Build history of the part. All positions in model axes, mm. Face numbers are marked on the shaded views. A direction names the side the tool comes from. Coordinates: 2 decimals unless noted, no trailing zeros. Order: outer loops, then holes, each group sorted by start corner. A loop starts at its lowest first (then second) coordinate and runs counter-clockwise, first axis right, second up. Notation, with made-up numbers: M 31,21.5 L 80,21.5 A12 cw 80,26.5 Z; hole C 27,87 d9. An arc over 180 degrees is marked long. Write item = value, one per line. Start each with the question number.
Q1. Band-saw the part on D-D on z = -35. Write the cut outline in (x, y), plus the area to 3 significant figures.
Q2. Band-saw the part on A-A on z = 0. Write the cut outline in (x, y), plus the area to 3 significant figures.
Q3. Pin check, flat tips, straight feed: P1, Ø5, axis at x = -102.5, z = 0, coming from the +Y side; P2, Ø1, axis at x = -105, y = -36, coming from the -Z side; P3, Ø6, axis at x = -121.5, y = -16.5, coming from the +Z side. Stop position of each tip, or through.
Q4. Drill centre lines: probe 1 along Y at (x, z) = (-73.5, 0); probe 2 along Y at (x, z) = (-113, 0); probe 3 along X at (y, z) = (-11, -49.5). Where is each one in solid material? Low to high.
Q5. Band-saw the part on B-B on y = 0. Write the cut outline in (x, z).
Q6. Pull direction Y, two halves, no side cores. Call the marked faces 1, 2 and 3: released by +Y, released by -Y, zero draft, split by the parting line, or undercut.
Q7. 3-axis set-ups, long thin cutter, end or side, ignore diameter. For the marked faces 4 and 5: which of +Z, -Z, +X, -X, +Y, -Y reach the whole face in a straight line?
Q8. Band-saw the part on C-C on x = -163. Write the cut outline in (y, z).
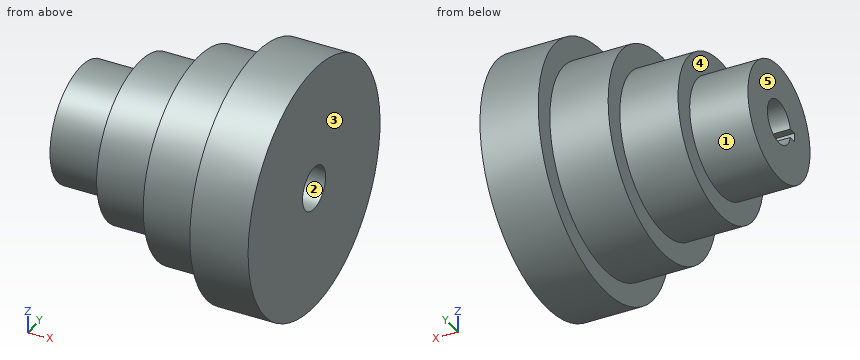
```python
from build123d import *

# Parameters (mm, degrees)
SKETCH2_W          = 6
SKETCH2_H          = 10
CUT_EXTRUDE3_DEPTH = 100


with BuildPart() as part:
    # Sketch1 → Revolve2 (revolve)
    with BuildSketch(Plane.XY, mode=Mode.PRIVATE) as revolve2_sk:
        Polygon((-45.142857143, 22.857142857), (-176, 22.857142857), (-176, 14.867713129), (-16, 14.867713129), (-16, 22.857142857), align=None)
        Polygon((-136, 40), (-176, 40), (-176, 22.857142857), (-45.142857143, 22.857142857), (-45.142857143, 37.142857143), (-128, 37.142857143), (-128, 47), (-88, 47), (-88, 62), (-48, 62), (-48, 77), (-16, 77), (-16, 85), (-56, 85), (-56, 70), (-96, 70), (-96, 55), (-136, 55), align=None)
        Polygon((-45.142857143, 37.142857143), (-45.142857143, 22.857142857), (-16, 22.857142857), (-16, 77), (-48, 77), (-48, 62), (-88, 62), (-88, 47), (-128, 47), (-128, 37.142857143), align=None)
    revolve(revolve2_sk.sketch.rotate(Axis((-176, 0, 0), (1, 0, 0)), 90), axis=Axis((-176, 0, 0), (1, 0, 0)))

    # Sketch2 → Cut-Extrude3 (cut)
    with BuildSketch(Plane.ZY.offset(176)):
        with Locations((0, -14.867713129)):
            Rectangle(SKETCH2_W, SKETCH2_H)
    extrude(amount=-CUT_EXTRUDE3_DEPTH, mode=Mode.SUBTRACT)


solid = part.part
```
Recorded:
q1.outline = M -176,-19.36 L -136,-19.36 L -136,-42.43 L -96,-42.43 L -96,-60.62 L -56,-60.62 L -56,-77.46 L -16,-77.46 L -16,77.46 L -56,77.46 L -56,60.62 L -96,60.62 L -96,42.43 L -136,42.43 L -136,19.36 L -176,19.36 Z
q1.area = 16,000 mm2
q2.outline = M -176,-40 L -136,-40 L -136,-55 L -96,-55 L -96,-70 L -56,-70 L -56,-85 L -16,-85 L -16,-14.87 L -76,-14.87 L -76,-19.87 L -176,-19.87 Z; M -176,14.87 L -16,14.87 L -16,85 L -56,85 L -56,70 L -96,70 L -96,55 L -136,55 L -136,40 L -176,40 Z
q2.area = 14,700 mm2
q3.P1 = 55
q3.P2 = -42.01
q3.P3 = 53.32
q4.probe_1 = -70 to -14.87, 14.87 to 70
q4.probe_2 = -55 to -19.87, 14.87 to 55
q4.probe_3 = -136 to -16
q5.outline = M -176,-40 L -136,-40 L -136,-55 L -96,-55 L -96,-70 L -56,-70 L -56,-85 L -16,-85 L -16,-14.87 L -176,-14.87 Z; M -176,14.87 L -16,14.87 L -16,85 L -56,85 L -56,70 L -96,70 L -96,55 L -136,55 L -136,40 L -176,40 Z
q6.face_1 = split by the parting line
q6.face_2 = undercut
q6.face_3 = zero draft
q7.face_4 = -X
q7.face_5 = +Z, -Z, -X, +Y, -Y
q8.outline = C 0,0 d80; hole M -19.87,-3 L -14.56,-3 A14.87 ccw long -14.56,3 L -19.87,3 Z
